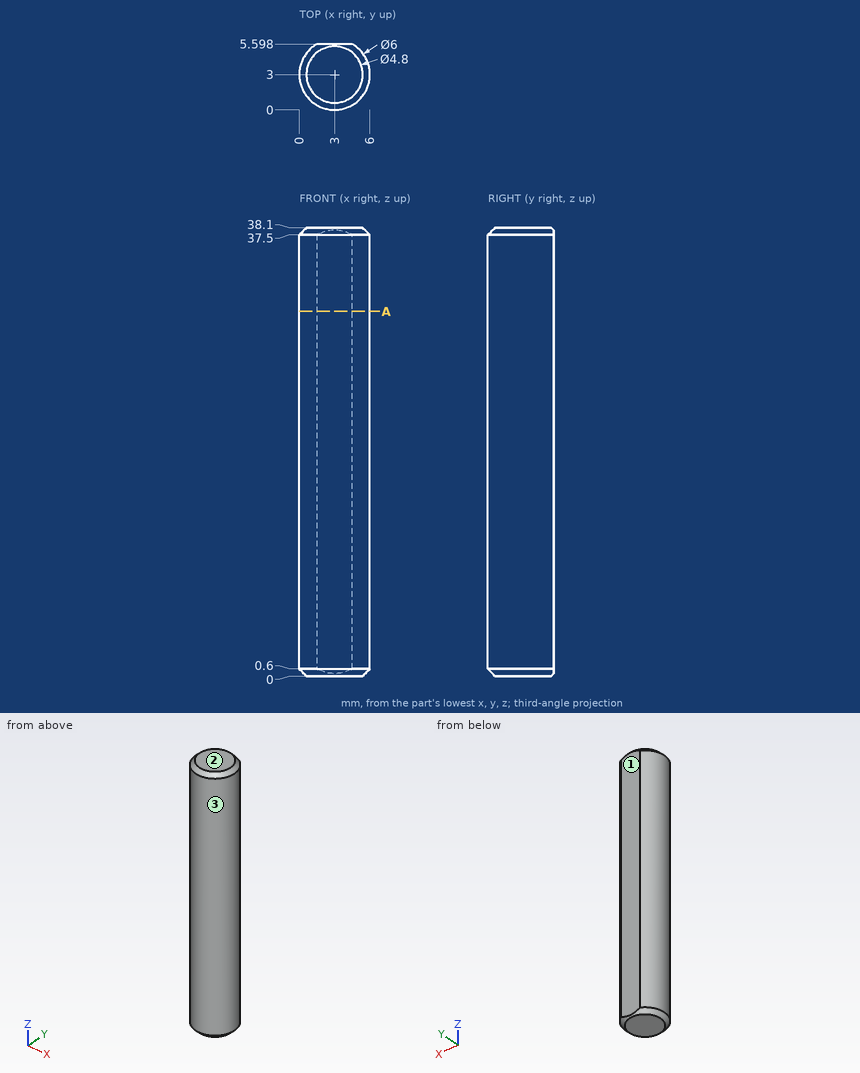
Here's the drawing with two shaded views (mm, measured from the low corner). I have some questions. Give positions to 0.01 mm unless a question says otherwise; leave off trailing zeros. Loops run counter-clockwise (first coordinate to the right, second up) from the corner with the lowest first, then second, coordinate; pieces in that order, holes last. Notation, with made-up numbers: M -2.5,68 L 50.5,68 A26 ccw 50.5,88 Z; hole C -17,6 d4. An arc over 180 degrees is marked long. Answer in a Markdown table with one row per item.
1. Suppose I cut it at A-A on z = 31. Write out the boundary of the cut face in (x, y), plus the area to 3 significant figures.
Taken from the geometry:
| item | result |
|---|---|
| outline | M 1.5,5.6 A3 ccw long 4.5,5.6 Z |
| area | 27.5 mm² |
2. For pin 1 Ø1 at (x, z) = (0.5, 29.5) entering from -Y; pin 2 Ø1.5 at (y, z) = (0.5, 32.5) entering from +X, each with a flat end and sliding along its axis, tell me the tip position at first contact or that it passes through.
Taken from the geometry:
| item | result |
|---|---|
| pin 1 | stops at y = 0.76 |
| pin 2 | stops at x = 5.44 |
3. If I drill on line 1 along Y through (x, z) = (3.1, 36); line 2 along Y through (x, z) = (5.6, 22); line 3 along X through (y, z) = (0.35, 10), over which ranges is the centre line in solid material (lowest first)?
Taken from the geometry:
| item | result |
|---|---|
| line 1 | y = 0 to 5.6 |
| line 2 | y = 1.5 to 4.5 |
| line 3 | x = 1.59 to 4.41 |
4. Thinking about a two-plate mould opening in Y: for the marked faces 1, 2 and 3, which applies, released by +Y, released by -Y, zero draft, split by the parting line, or undercut?
Taken from the geometry:
| item | result |
|---|---|
| face 1 | released by +Y |
| face 2 | zero draft |
| face 3 | split by the parting line |
